Answer from the drawing. Dimensions are ordinates in mm from the lowest x, y and z of the part. A direction names the side the tool comes from. Round coordinates to 2 decimals unless told otherwise and drop trailing zeros. Loops run counter-clockwise (first coordinate to the right, second up) from the corner with the lowest first, then second, coordinate; pieces in that order, holes last. Notation, with made-up numbers: M -35.5,-37.75 L -9.5,-37.75 A6 ccw -9.5,-27.75 Z; hole C 40,-11 d11. An arc over 180 degrees is marked long. Answer as CSV lines item,"result".
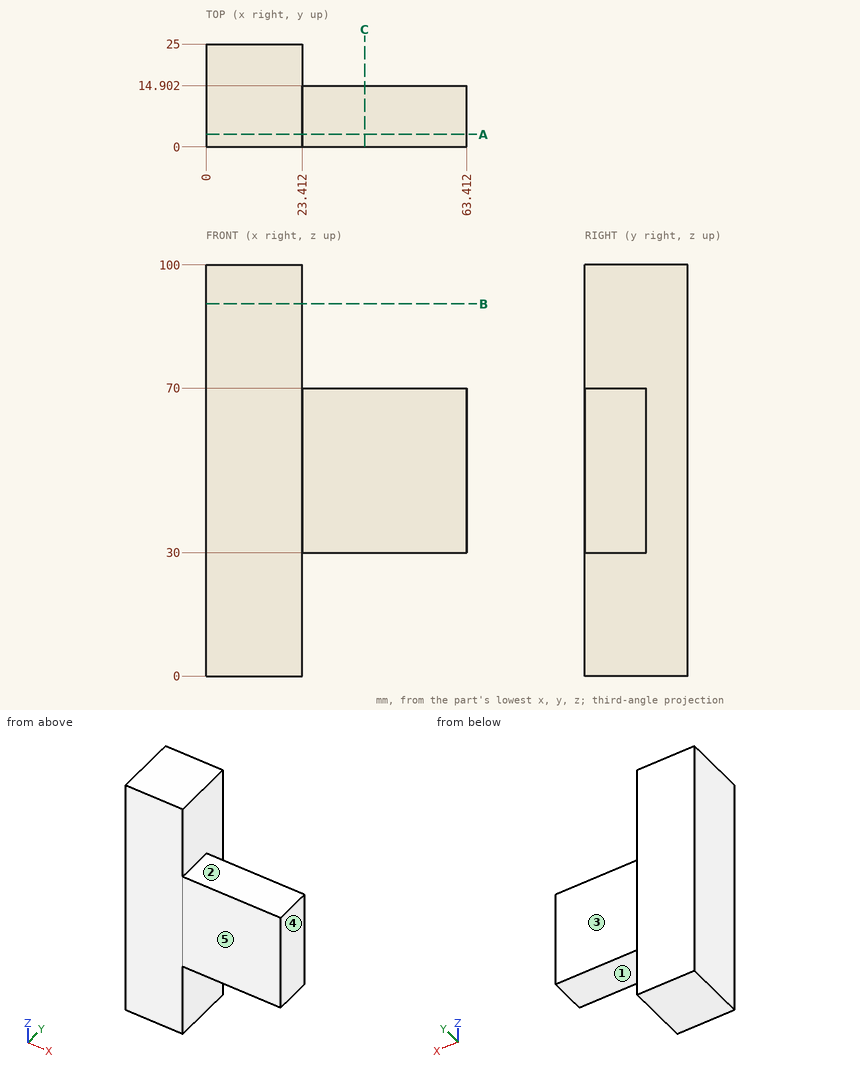
1) Find section B-B, the plane z = 90.5. Give the vertices of the cut face in (x, y).
Evaluation:
outline,"M 0,0 L 23.41,0 L 23.41,25 L 0,25 Z"
2) Find section A-A, the plane y = 3. Give the vertices of the cut face in (x, z).
Evaluation:
outline,"M 0,0 L 23.41,0 L 23.41,30 L 63.41,30 L 63.41,70 L 23.41,70 L 23.41,100 L 0,100 Z"
3) Straight lines are drawn through the part: line 1 (X direction, y = 11, z = 80); line 2 (Z direction, x = 23.5, y = 13); line 3 (Y direction, x = 44, z = 44.5). For each, find the intervals that lie inside material, in ascending order.
Evaluation:
line 1,"x = 0 to 23.41"
line 2,"z = 30 to 70"
line 3,"y = 0 to 14.9"
4) Find section C-C, the plane x = 38.5. Give the vertices of the cut face in (y, z).
Evaluation:
outline,"M 0,30 L 14.9,30 L 14.9,70 L 0,70 Z"
5) Each of these flat-tipped pins is pushed along its axis until it touches: P1, Ø8, axis at x = 28, z = 67.5, coming from the -Y side; P2, Ø4, axis at x = 52, z = 34, coming from the +Y side; P3, Ø12, axis at x = 37, y = 8, coming from the +Z side. Where does it stop, or does it pass through?
Evaluation:
P1,"stops at y = 0"
P2,"stops at y = 14.9"
P3,"stops at z = 70"
6) A tool of negligible diameter and unlimited length cuts with its end or side. For the marked faces 1, 2, 3, 4 and 5, from which of +Z, -Z, +X, -X, +Y, -Y can it reach the whole face along a straight path? Write none if from no direction.
Evaluation:
face 1,"-Z, +X, +Y, -Y"
face 2,"+Z, +X, +Y, -Y"
face 3,"+Z, -Z, +X, +Y"
face 4,"+Z, -Z, +X, +Y, -Y"
face 5,"+Z, -Z, +X, -X, -Y"
